Check sheet for the drawn part. Datum: minimum x, y, z corner. Units: mm. A direction names the side the tool comes from. Round coordinates to 2 decimals unless told otherwise and drop trailing zeros. Order: outer loops, then holes, each group sorted by start corner. A loop starts at its lowest first (then second) coordinate and runs counter-clockwise, first axis right, second up. Notation, with made-up numbers: (5.5, -9) -> (28.5, -9) arc R16 cw to (28.5, -1) -> close; hole circle Ø5 at (-38, -18). An arc over 180 degrees is marked (long way). Answer in a Markdown table with one row per item.
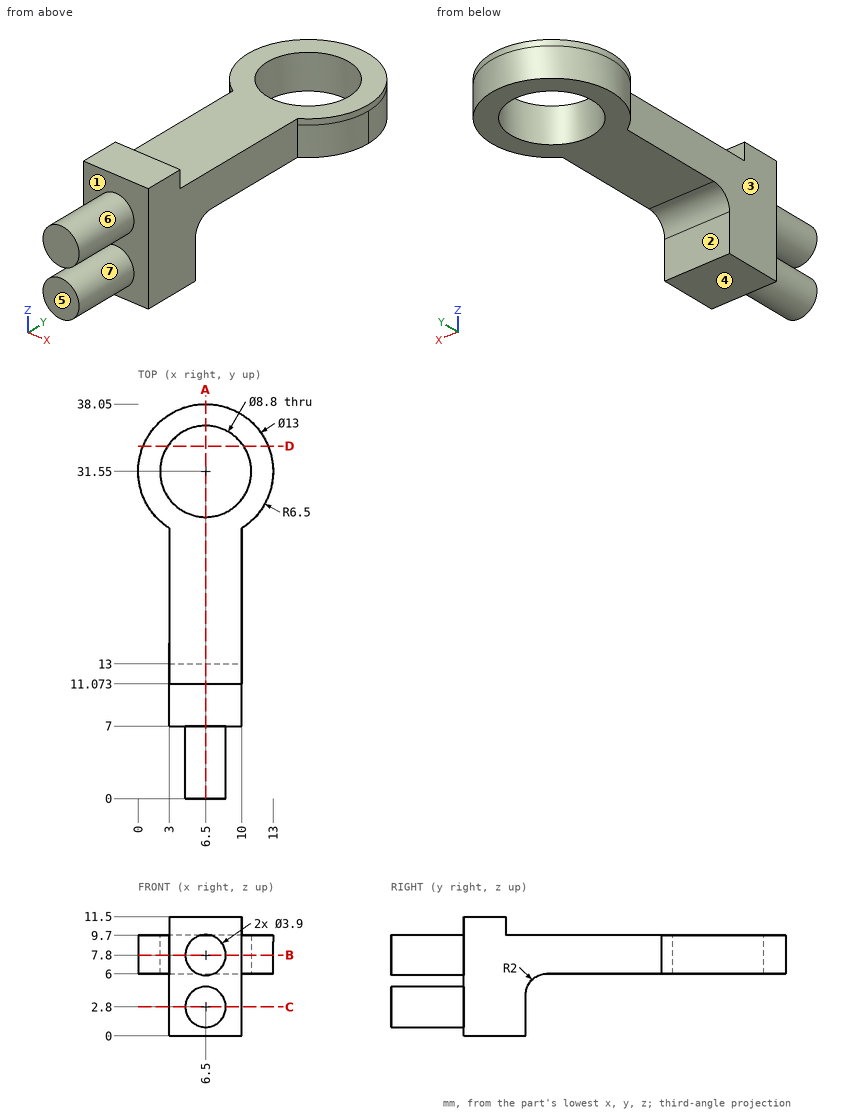
(1) Section check B-B on z = 7.8. Record the boundary of the cut face in (x, y).
Solutions:
| item | result |
|---|---|
| outline | (3, 7) -> (4.55, 7) -> (4.55, 0) -> (8.45, 0) -> (8.45, 7) -> (10, 7) -> (10, 26.07) arc R6.5 ccw (long way) to (3, 26.07) -> close; hole circle Ø8.8 at (6.5, 31.55) |
(2) Depth check by flat-ended pin: pin 1 Ø1.4 at (x, z) = (7.5, 10.5) entering from +Y; pin 2 Ø5 at (y, z) = (14.5, 6) entering from -X; pin 3 Ø6.5 at (x, y) = (3.5, 29.5) entering from -Z; pin 4 Ø5.5 at (x, y) = (6.5, 31.55) entering from +Z. Enter the tip coordinate at first touch or a pass-through.
Solutions:
| item | result |
|---|---|
| pin 1 | y = 11.07 |
| pin 2 | x = 3 |
| pin 3 | z = 6 |
| pin 4 | through |
(3) Section check C-C on z = 2.8. Record the boundary of the cut face in (x, y), plus the area to 3 significant figures.
Solutions:
| item | result |
|---|---|
| outline | (3, 7) -> (4.55, 7) -> (4.55, 0) -> (8.45, 0) -> (8.45, 7) -> (10, 7) -> (10, 13) -> (3, 13) -> close |
| area | 69.3 mm^2 |
(4) Draft check along Z on the marked faces 4, 5, 6 and 7. Enter one of: pulls with the +Z half, pulls with the -Z half, needs draft (parallel to the pull), parting line crosses it, or undercut.
Solutions:
| item | result |
|---|---|
| face 4 | pulls with the -Z half |
| face 5 | needs draft |
| face 6 | undercut |
| face 7 | undercut |
(5) Tool access check on the marked faces 1, 2 and 3. Record the directions out of +Z, -Z, +X, -X, +Y, -Y that give a thin tool (end or side, any length) a straight path to the whole face; none if there is none.
Solutions:
| item | result |
|---|---|
| face 1 | -Y |
| face 2 | -Z, +X, -X, +Y |
| face 3 | +Z, -Z, -X, -Y |
(6) Section check A-A on x = 6.5. Record the boundary of the cut face in (y, z), plus the area to 3 significant figures.
Solutions:
| item | result |
|---|---|
| outline | (0, 0.85) -> (7, 0.85) -> (7, 0) -> (13, 0) -> (13, 4) arc R2 cw to (15, 6) -> (27.15, 6) -> (27.15, 9.7) -> (11.07, 9.7) -> (11.07, 11.5) -> (7, 11.5) -> (7, 9.75) -> (0, 9.75) -> (0, 5.85) -> (7, 5.85) -> (7, 4.75) -> (0, 4.75) -> close; (35.95, 6) -> (38.05, 6) -> (38.05, 9.7) -> (35.95, 9.7) -> close |
| area | 181 mm^2 |
(7) Section check D-D on y = 34. Record the boundary of the cut face in (x, z) (1 decimal).
Solutions:
| item | result |
|---|---|
| outline | (0.5, 6) -> (2.8, 6) -> (2.8, 9.7) -> (0.5, 9.7) -> close; (10.2, 6) -> (12.5, 6) -> (12.5, 9.7) -> (10.2, 9.7) -> close |
(8) Scan lines: probe 1 along Y at (x, z) = (6.25, 7.5) (1 decimal); probe 2 along Z at (x, y) = (8, 3.5) (1 decimal); probe 3 along X at (y, z) = (26, 6.75). Record each from-to range of solid material in increasing order. Write a range as from..to.
Solutions:
| item | result |
|---|---|
| probe 1 | 0..27.2, 35.9..38 |
| probe 2 | 1.6..4, 6.6..9 |
| probe 3 | 3..10 |
